Verification items for the finished model (mm, model axes). Face numbers are marked on the shaded views. Round coordinates to 2 decimals unless told otherwise and drop trailing zeros. Loops run counter-clockwise (first coordinate to the right, second up) from the corner with the lowest first, then second, coordinate; pieces in that order, holes last. Notation, with made-up numbers: (-6, 11) -> (51, 11) arc R6 cw to (51, 18) -> close; hole circle Ø4 at (34, 76). An arc over 180 degrees is marked (long way). Use a Markdown table: item, result. Add a question column.
```python
from build123d import *

# Parameters (mm, degrees)
SKETCH_1_R          = 24.85
SKETCH_1_R_2        = 2.25
EXTRUDE_1_DEPTH     = 7.5
SKETCH_3_R          = 27.5
SKETCH_3_R_2        = 24.85
EXTRUDE_2_DEPTH     = 2.8
SKETCH_4_R          = 10
CUT_EXTRUDE_1_DEPTH = 40.607448794


with BuildPart() as part:
    # 草图1 → 凸台-拉伸1 (new body)
    with BuildSketch(Plane.XY):
        Circle(SKETCH_1_R)
        with Locations((-21.75, 0)):
            Circle(SKETCH_1_R_2, mode=Mode.SUBTRACT)
        with Locations((-13.980630511, 16.661466638)):
            Circle(SKETCH_1_R_2, mode=Mode.SUBTRACT)
        with Locations((-13.980630511, -16.661466638)):
            Circle(SKETCH_1_R_2, mode=Mode.SUBTRACT)
        with Locations((13.980630511, -16.661466638)):
            Circle(SKETCH_1_R_2, mode=Mode.SUBTRACT)
        with Locations((21.75, 0)):
            Circle(SKETCH_1_R_2, mode=Mode.SUBTRACT)
        with Locations((13.980630511, 16.661466638)):
            Circle(SKETCH_1_R_2, mode=Mode.SUBTRACT)
    extrude(amount=EXTRUDE_1_DEPTH)

    # 草图3 → 凸台-拉伸2 (add)
    with BuildSketch(Plane.XY):
        Circle(SKETCH_3_R)
        Circle(SKETCH_3_R_2, mode=Mode.SUBTRACT)
    extrude(amount=EXTRUDE_2_DEPTH)

    # 草图4 → 切除-拉伸1 (cut, through all)
    with BuildSketch(Plane(origin=(0, 0, 0), x_dir=(-1, 0, 0), z_dir=(0, 0, -1))):
        Circle(SKETCH_4_R)
    extrude(amount=-CUT_EXTRUDE_1_DEPTH, mode=Mode.SUBTRACT)


solid = part.part
```
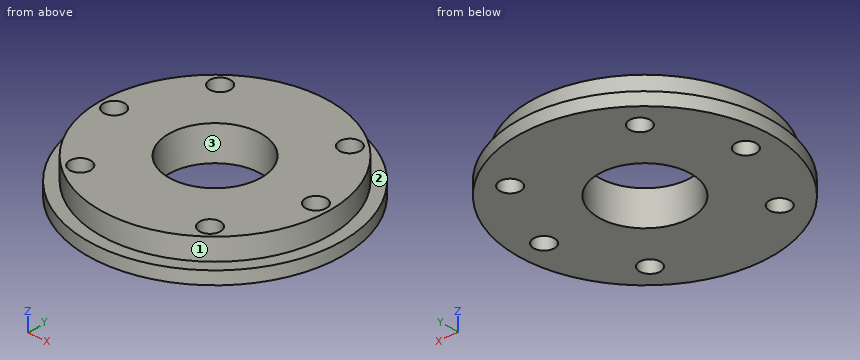
1) Go/stop test with flat-tipped pins: pin 1 (1 mm diameter, centred on x = 16, z = 5, fed in from -Y); pin 2 (3.5 mm diameter, centred on x = -13.98, y = -16.66, fed in from -Z). Record where each tip stops, or that it passes through.
2) Sectioned sample at C-C on y = 5.5. Enter the section's corners in (x, z), then the cut area to 3 significant figures.
3) Release check for a two-part mould opening along X. For the marked faces 1, 2 and 3 record: released by +X, released by -X, zero draft, split by the parting line, or undercut.
4) Sectioned sample at D-D on z = 1.25. Enter the section's corners in (x, y).
5) Sectioned sample at B-B on y = 0. Enter the section's corners in (x, z), then the cut area to 3 significant figures.
6) Thickness scan on line 1 (X direction, y = -17.5, z = 5.5); line 2 (Y direction, x = -12, z = 4); line 3 (Y direction, x = -15, z = 4). Record the ranges inside material, lowest first.
7) Sectioned sample at A-A on x = 0. Enter the section's corners in (y, z), then the cut area to 3 significant figures.
Geometry results:
| question | item | result |
|---|---|---|
| 1 | pin 1 | y = -19.42 |
| 1 | pin 2 | through |
| 2 | outline | (-26.94, 0) -> (-8.35, 0) -> (-8.35, 7.5) -> (-24.23, 7.5) -> (-24.23, 2.8) -> (-26.94, 2.8) -> close; (8.35, 0) -> (26.94, 0) -> (26.94, 2.8) -> (24.23, 2.8) -> (24.23, 7.5) -> (8.35, 7.5) -> close |
| 2 | area | 253 mm^2 |
| 3 | face 1 | split by the parting line |
| 3 | face 2 | zero draft |
| 3 | face 3 | undercut |
| 4 | outline | circle Ø55 at (0, 0); hole circle Ø4.5 at (-21.75, 0); hole circle Ø4.5 at (-13.98, -16.66); hole circle Ø4.5 at (-13.98, 16.66); hole circle Ø20 at (0, 0); hole circle Ø4.5 at (13.98, -16.66); hole circle Ø4.5 at (13.98, 16.66); hole circle Ø4.5 at (21.75, 0) |
| 5 | outline | (-27.5, 0) -> (-24, 0) -> (-24, 7.5) -> (-24.85, 7.5) -> (-24.85, 2.8) -> (-27.5, 2.8) -> close; (-19.5, 0) -> (-10, 0) -> (-10, 7.5) -> (-19.5, 7.5) -> close; (10, 0) -> (19.5, 0) -> (19.5, 7.5) -> (10, 7.5) -> close; (24, 0) -> (27.5, 0) -> (27.5, 2.8) -> (24.85, 2.8) -> (24.85, 7.5) -> (24, 7.5) -> close |
| 5 | area | 170 mm^2 |
| 6 | line 1 | -17.64 to -16.07, -11.89 to 11.89, 16.07 to 17.64 |
| 6 | line 2 | -21.76 to -17.73, -15.59 to 15.59, 17.73 to 21.76 |
| 6 | line 3 | -19.81 to -18.67, -14.66 to 14.66, 18.67 to 19.81 |
| 7 | outline | (-27.5, 0) -> (-10, 0) -> (-10, 7.5) -> (-24.85, 7.5) -> (-24.85, 2.8) -> (-27.5, 2.8) -> close; (10, 0) -> (27.5, 0) -> (27.5, 2.8) -> (24.85, 2.8) -> (24.85, 7.5) -> (10, 7.5) -> close |
| 7 | area | 238 mm^2 |
